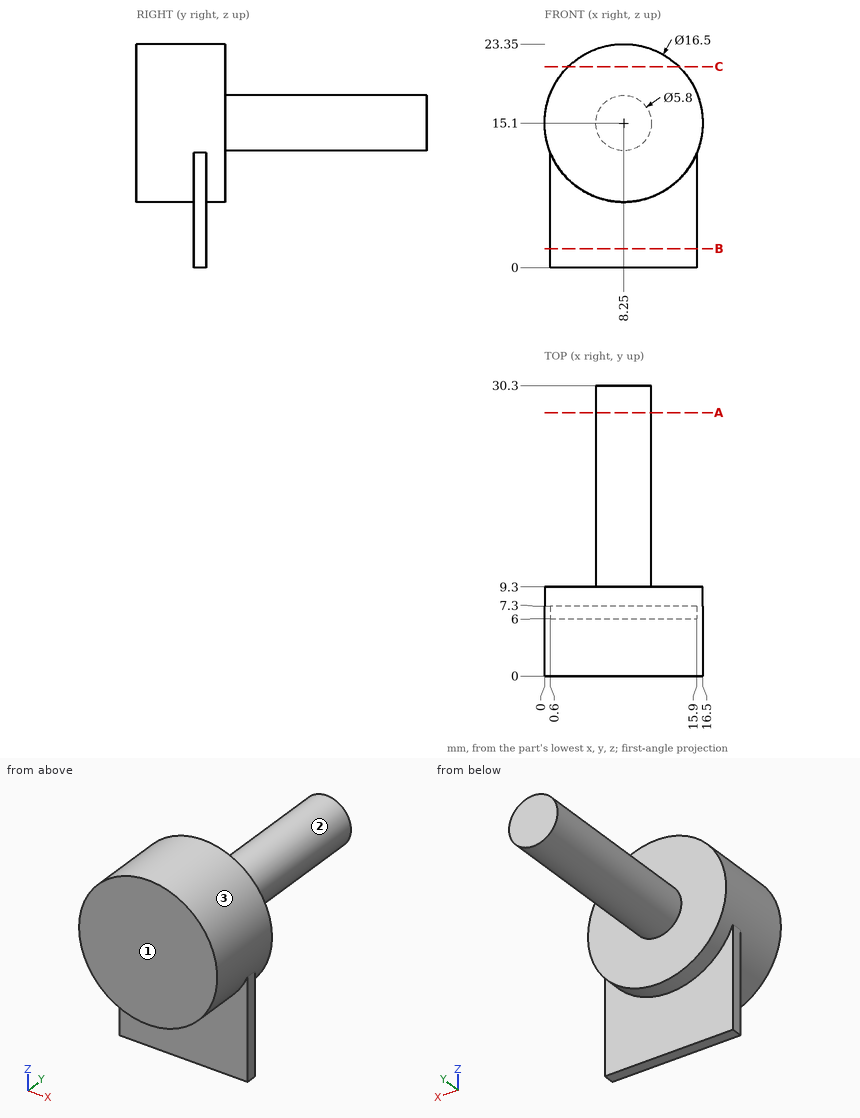
Geometry check sheet. Reference: drawing and pictorial views, mm from the part's lowest x, y, z. A direction names the side the tool comes from. Round coordinates to 2 decimals unless told otherwise and drop trailing zeros. Write each loop counter-clockwise with the first axis right and the second up, starting at its lowest first coordinate (ties: lowest second). Pieces come first, ordered by that corner, then holes. Notation, with made-up numbers: (88.5, 39.5) -> (92.5, 39.5) arc R11 ccw to (92.5, 56.5) -> close; hole circle Ø9 at (-21.75, 56). An arc over 180 degrees is marked (long way). One line per question, with ' | ' between items. Start each with the question number.
1. Sectioned sample at C-C, the plane z = 21. Record the cut outline in (x, y).
2. Scan lines: line 1 along Y through (x, z) = (3.5, 8); line 2 along Y through (x, z) = (12.25, 18.5); line 3 along X through (y, z) = (6.5, 9.5). Record each from-to range of solid material in increasing order. Write a range as from..to.
3. Sectioned sample at A-A, the plane y = 27.5. Record the cut outline in (x, z).
4. Depth check by flat-ended pin: pin 1 (8 mm diameter, centred on x = 10.5, y = 12.5, fed in from -Z); pin 2 (2 mm diameter, centred on x = 5, y = 8.5, fed in from -Z); pin 3 (1.5 mm diameter, centred on x = 10, y = 15, fed in from +Z); pin 4 (4 mm diameter, centred on x = 2, y = 12, fed in from -Z). Enter the tip coordinate at first touch or a pass-through.
5. Sectioned sample at B-B, the plane z = 2. Record the cut outline in (x, y), then the cut area to 3 significant figures.
6. Set-up check for the marked faces 1, 2 and 3: record each of +Z, -Z, +X, -X, +Y, -Y from which the full face is reachable in a straight line by a thin tool's end or side.
Taken from the geometry:
1) outline: (2.48, 0) -> (14.02, 0) -> (14.02, 9.3) -> (2.48, 9.3) -> close
2) line 1: y = 6..7.3 | line 2: y = 0..9.3 | line 3: x = 0.6..15.9
3) outline: circle Ø5.8 at (8.25, 15.1)
4) pin 1: stops at z = 6.85 | pin 2: stops at z = 7.16 | pin 3: stops at z = 17.82 | pin 4: passes through
5) outline: (0.6, 6) -> (15.9, 6) -> (15.9, 7.3) -> (0.6, 7.3) -> close | area: 19.9 mm^2
6) face 1: +Z, -Z, +X, -X, -Y | face 2: +Y | face 3: none
